Answer from the drawing. Dimensions are ordinates in mm from the lowest x, y and z of the part. Round coordinates to 2 decimals unless told otherwise and drop trailing zeros. Loops run counter-clockwise (first coordinate to the right, second up) from the corner with the lowest first, then second, coordinate; pieces in that order, holes last. Notation, with made-up numbers: (55, 27) - (99, 27) arc R13 ccw to (99, 33) - close; hole circle Ø9 at (-2.75, -32.5). An arc over 180 degrees is marked (long way). Return JSON: item names as keys, results as strings.
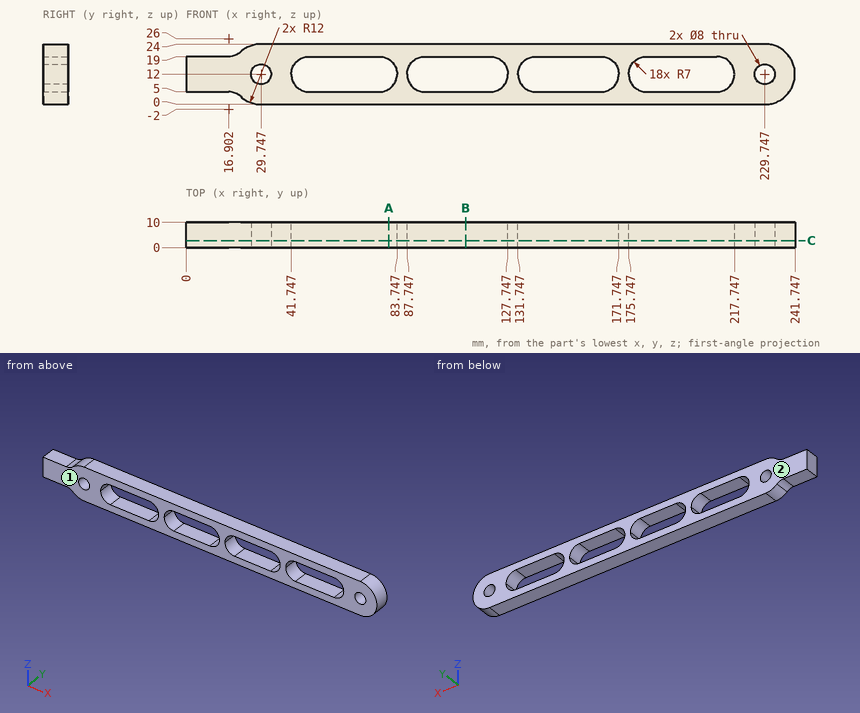
1) Section B-B (x = 111) is taken. Give the vertices of the cut face in (y, z), and give its area (3 significant figures).
Verdict:
{"outline": "(0, 0) - (10, 0) - (10, 5) - (0, 5) - close; (0, 19) - (10, 19) - (10, 24) - (0, 24) - close", "area": "100 mm2"}
2) Determine the mould class of the marked faces 1 and 2 for opening direction Y: pulls with the +Y half, pulls with the -Y half, needs draft (parallel to the pull), parting line crosses it, or undercut.
Verdict:
{"face 1": "pulls with the -Y half", "face 2": "pulls with the +Y half"}
3) Section A-A (x = 80.5) is taken. Give the vertices of the cut face in (y, z).
Verdict:
{"outline": "(0, 0) - (10, 0) - (10, 6.09) - (0, 6.09) - close; (0, 17.91) - (10, 17.91) - (10, 24) - (0, 24) - close"}
4) Find the intervals of material crossed by L1, parallel to Z at x = 100.5, y = 5.5; L2, parallel to Z at x = 30, y = 1.25; L3, parallel to X at y = 3.25, z = 22.5 (1 decimal), in increasing order.
Verdict:
{"L1": "z = 0 to 5, 19 to 24", "L2": "z = 0 to 8.01, 15.99 to 24", "L3": "x = 23.9 to 235.6"}
5) A flat-ended cylindrical pin translates along its axis: pin 1 (6 mm diameter, centred on y = 5.5, z = 17.5, fed in from +X). Find the tip coordinate at first contact, or state that the pin passes through.
Verdict:
{"pin 1": "stops at x = 241.48"}
6) Section C-C (y = 2.75) is taken. Count the separate pieces of the cut face and the enclosed holes in it.
Verdict:
{"separate pieces": "1", "enclosed holes": "6"}
